Geometry check sheet. Reference: drawing and pictorial views, mm from the part's lowest x, y, z. A direction names the side the tool comes from. Give positions to 0.01 mm unless a question says otherwise; leave off trailing zeros. Write each loop counter-clockwise with the first axis right and the second up, starting at its lowest first coordinate (ties: lowest second). Pieces come first, ordered by that corner, then holes. Notation, with made-up numbers: (-26, 65) -> (-10, 65) arc R9 ccw to (-10, 73) -> close; hole circle Ø2 at (12.5, 81.25). An arc over 180 degrees is marked (long way). Answer as CSV lines item,"result".
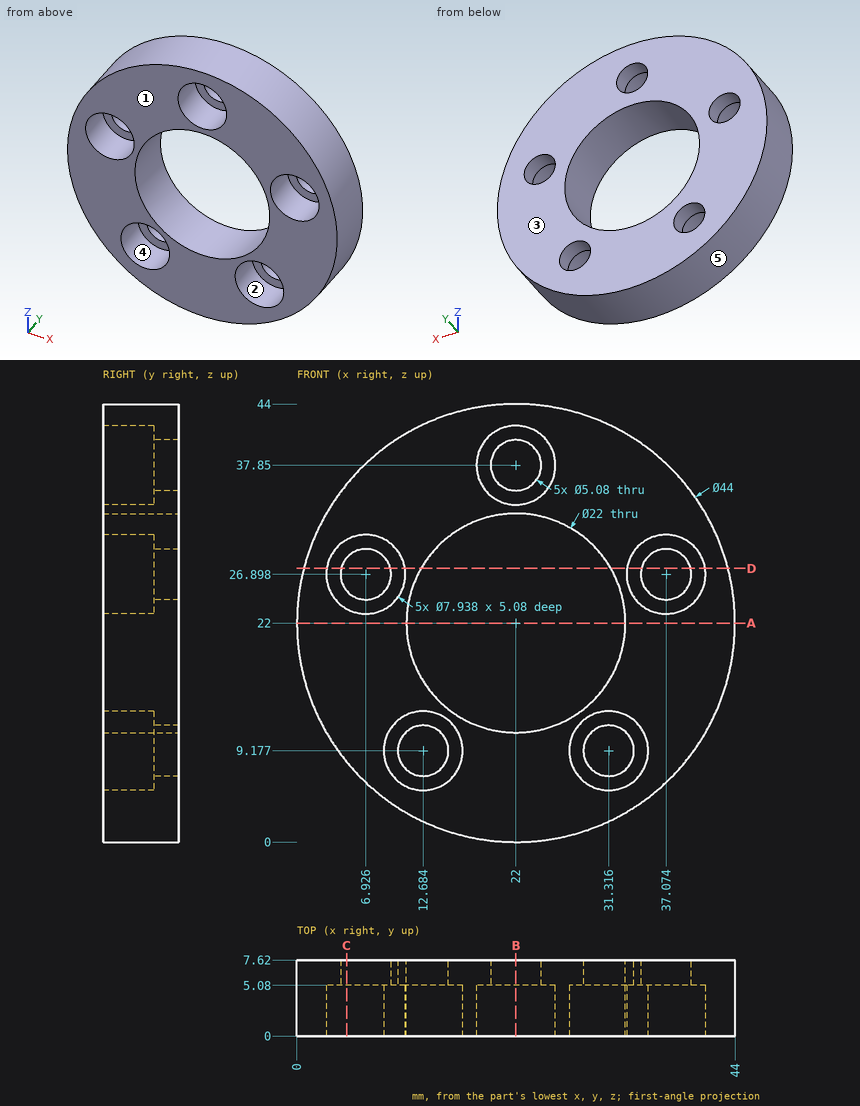
1) Section check D-D (z = 27.5). Record the boundary of the cut face in (x, y).
Reported:
outline,"(0.7, 0) -> (3, 0) -> (3, 5.08) -> (4.46, 5.08) -> (4.46, 7.62) -> (0.7, 7.62) -> close; (9.39, 5.08) -> (10.85, 5.08) -> (10.85, 0) -> (12.47, 0) -> (12.47, 7.62) -> (9.39, 7.62) -> close; (31.53, 0) -> (33.15, 0) -> (33.15, 5.08) -> (34.61, 5.08) -> (34.61, 7.62) -> (31.53, 7.62) -> close; (39.54, 5.08) -> (41, 5.08) -> (41, 0) -> (43.3, 0) -> (43.3, 7.62) -> (39.54, 7.62) -> close"
2) Tool access check on the marked faces 1 and 2. Record the directions out of +Z, -Z, +X, -X, +Y, -Y that give a thin tool (end or side, any length) a straight path to the whole face; none if there is none.
Reported:
face 1,"+Z, -Z, +X, -X, -Y"
face 2,"-Y"
3) Section check B-B (x = 22). Record the boundary of the cut face in (y, z), and give its area (3 significant figures).
Reported:
outline,"(0, 0) -> (7.62, 0) -> (7.62, 11) -> (0, 11) -> close; (0, 33) -> (7.62, 33) -> (7.62, 35.31) -> (5.08, 35.31) -> (5.08, 33.88) -> (0, 33.88) -> close; (0, 41.82) -> (5.08, 41.82) -> (5.08, 40.39) -> (7.62, 40.39) -> (7.62, 44) -> (0, 44) -> close"
area,"114 mm²"
4) Section check C-C (x = 5). Record the boundary of the cut face in (y, z) (1 decimal), and give its area (3 significant figures).
Reported:
outline,"(0, 8) -> (7.6, 8) -> (7.6, 25.2) -> (5.1, 25.2) -> (5.1, 23.4) -> (0, 23.4) -> close; (0, 30.4) -> (5.1, 30.4) -> (5.1, 28.6) -> (7.6, 28.6) -> (7.6, 36) -> (0, 36) -> close"
area,"169 mm²"
5) Section check A-A (z = 22). Record the boundary of the cut face in (x, y), and give its area (3 significant figures).
Reported:
outline,"(0, 0) -> (11, 0) -> (11, 7.62) -> (0, 7.62) -> close; (33, 0) -> (44, 0) -> (44, 7.62) -> (33, 7.62) -> close"
area,"168 mm²"
6) Depth check by flat-ended pin: pin 1 (5 mm diameter, centred on x = 24, z = 29, fed in from +Y); pin 2 (4 mm diameter, centred on x = 20.5, z = 37.5, fed in from -Y); pin 3 (2 mm diameter, centred on x = 20.5, y = 4.5, fed in from -Z). Enter the tip coordinate at first touch or a pass-through.
Reported:
pin 1,"through"
pin 2,"y = 5.08"
pin 3,"z = 0.01"
7) Scan lines: line 1 along Z through (x, y) = (21.5, 4.25) (1 decimal); line 2 along Z through (x, y) = (24, 1) (1 decimal); line 3 along Z through (x, y) = (27, 2.5) (1 decimal). Record each from-to range of solid material in increasing order.
Reported:
line 1,"0 to 11, 33 to 33.9, 41.8 to 44"
line 2,"0.1 to 11.2, 32.8 to 34.4, 41.3 to 43.9"
line 3,"0.6 to 12.2, 31.8 to 43.4"
8) Draft check along X on the marked faces 3, 4 and 5. Enter one of: +X half, -X half, draft (parallel to the pull), parting line (faces both ways), or undercut.
Reported:
face 3,"draft"
face 4,"undercut"
face 5,"parting line"
